Work out the finished part from the listing and answer in its coordinate system (mm). Face numbers are marked on the shaded views. A direction names the side the tool comes from. Give positions to 0.01 mm unless a question says otherwise; leave off trailing zeros. Loops run counter-clockwise (first coordinate to the right, second up) from the corner with the lowest first, then second, coordinate; pieces in that order, holes last. Notation, with made-up numbers: (11.25, -10) - (51.25, -10) arc R17 ccw to (51.25, -6) - close; hole circle Ø9 at (-11, 65.5). An arc over 180 degrees is marked (long way). Use CSV: the item, a comma, the result in double quotes.
from build123d import *

# Parameters (mm, degrees)
SKETCH1_W           = 222.25
SKETCH1_H           = 60.325
BOSS_EXTRUDE1_DEPTH = 25.4
SKETCH2_W           = 12.7
SKETCH2_H           = 60.325
BOSS_EXTRUDE2_DEPTH = 1.5875
SKETCH3_R           = 1.5875
CUT_EXTRUDE1_DEPTH  = 2.5875
SKETCH4_W           = 4.7625
SKETCH4_H           = 19.05
BOSS_EXTRUDE3_DEPTH = 5.08
SKETCH5_W           = 15.875
SKETCH5_H           = 7.9375
BOSS_EXTRUDE4_DEPTH = 12.7
LPATTERN1_COUNT     = 5
LPATTERN1_PITCH     = 22.86
LPATTERN1_COL_COUNT = 5
LPATTERN1_COL_PITCH = 22.86


with BuildPart() as part:
    # Sketch1 → Boss-Extrude1 (new body)
    with BuildSketch(Plane(origin=(0, 0, 0), x_dir=(1, 0, 0), z_dir=(0, 1, 0))):
        with Locations((111.125, 30.1625)):
            Rectangle(SKETCH1_W, SKETCH1_H)
    extrude(amount=BOSS_EXTRUDE1_DEPTH)

    # Sketch2 → Boss-Extrude2 (add)
    with BuildSketch(Plane.XZ):
        with Locations((228.6, -30.1625)):
            Rectangle(SKETCH2_W, SKETCH2_H)
        with Locations((-6.35, -30.1625)):
            Rectangle(SKETCH2_W, SKETCH2_H)
    extrude(amount=-BOSS_EXTRUDE2_DEPTH)

    # Sketch3 → Cut-Extrude1 (cut, through all)
    with BuildSketch(Plane(origin=(0, 1.5875, 0), x_dir=(1, 0, 0), z_dir=(0, 1, 0))):
        with Locations((-7.9375, 46.0375)):
            Circle(SKETCH3_R)
        with Locations((-7.9375, 14.2875)):
            Circle(SKETCH3_R)
        with Locations((230.1875, 14.2875)):
            Circle(SKETCH3_R)
        with Locations((230.1875, 46.0375)):
            Circle(SKETCH3_R)
    extrude(amount=-CUT_EXTRUDE1_DEPTH, mode=Mode.SUBTRACT)

    # Sketch4 → Boss-Extrude3 (add)
    with BuildSketch(Plane(origin=(0, 25.4, 0), x_dir=(1, 0, 0), z_dir=(0, 1, 0))):
        with Locations((111.125, 41.275)):
            Rectangle(SKETCH4_W, SKETCH4_H)
    boss_extrude3 = extrude(amount=BOSS_EXTRUDE3_DEPTH)

    # Sketch5 → Boss-Extrude4 (add)
    with BuildSketch(Plane.XY):
        with Locations((111.125, 13.49375)):
            Rectangle(SKETCH5_W, SKETCH5_H)
    boss_extrude4 = extrude(amount=BOSS_EXTRUDE4_DEPTH)

    # LPattern1: Boss-Extrude3, Boss-Extrude4 ×5
    with Locations(*[(i * LPATTERN1_PITCH, 0, 0) for i in range(1, LPATTERN1_COUNT)]):
        add(boss_extrude3)
        add(boss_extrude4)

    # LPattern1 col: Boss-Extrude3, Boss-Extrude4 ×5
    with Locations(*[(-i * LPATTERN1_COL_PITCH, 0, 0) for i in range(1, LPATTERN1_COL_COUNT)]):
        add(boss_extrude3)
        add(boss_extrude4)


solid = part.part
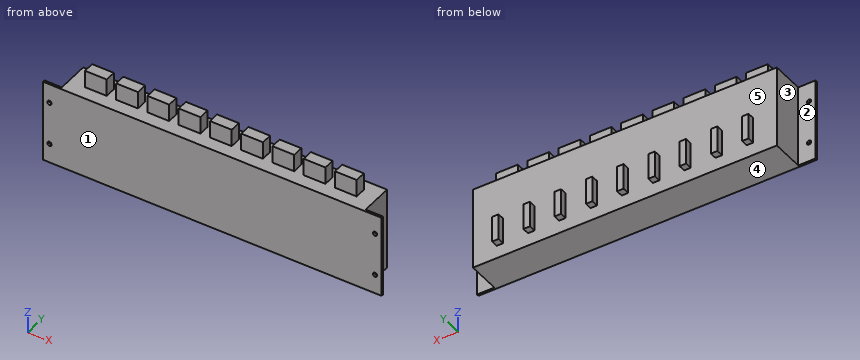
Item 1: A cutting plane is placed at D-D on z = 6. State how many separate pieces and enclosed holes the cut face has, and give its area (3 significant figures).
Determined:
separate pieces,"9"
enclosed holes,"0"
area,"1,130 mm²"
Item 2: A cutting plane is placed at A-A on z = -20.5. Determine the outline of the cut face in (x, y), and give its area (3 significant figures).
Determined:
outline,"(-12.7, 0) - (234.95, 0) - (234.95, 1.59) - (222.25, 1.59) - (222.25, 25.4) - (0, 25.4) - (0, 1.59) - (-12.7, 1.59) - close"
area,"5,690 mm²"
Item 3: For the marked faces 1 and 2, determine the directions among +Z, -Z, +X, -X, +Y, -Y from which every point of the face is accessible in a straight line to the end or side of a thin tool.
Determined:
face 1,"+Z, -Z, +X, -X, -Y"
face 2,"+Z, -Z, -X, +Y"
Item 4: A cutting plane is placed at C-C on y = 4. Determine the outline of the cut face in (x, z) (3 decimals), and give its area (3 significant figures).
Determined:
outline,"(0, -60.325) - (222.25, -60.325) - (222.25, 0) - (0, 0) - close"
area,"13,400 mm²"
Item 5: A cutting plane is placed at B-B on x = 207.5. Determine the outline of the cut face in (y, z) (1 decimal).
Determined:
outline,"(0, -60.3) - (25.4, -60.3) - (25.4, 0) - (17.5, 0) - (17.5, 12.7) - (9.5, 12.7) - (9.5, 0) - (0, 0) - close"
Item 6: Find the intervals of material crossed by line 1 (X direction, y = 20.5, z = -9.5); line 2 (Y direction, x = 27, z = -41); line 3 (Z direction, x = 190, y = 16) (3 decimals), in increasing order.
Determined:
line 1,"x = 0 to 222.25"
line 2,"y = 0 to 25.4"
line 3,"z = -60.325 to 0"
Item 7: Given P1, Ø2.5, axis at y = 27, z = -41, coming from the -X side; P2, Ø10, axis at x = 96, z = -8.5, coming from the +Y side; P3, Ø2.5, axis at y = 15, z = 8.5, coming from the -X side; P4, Ø8, axis at x = 121.5, y = 15.5, coming from the +Z side, each flat-ended and moving along its own axis, determine where each tip first touches the part or whether it passes through.
Determined:
P1,"stops at x = 17.3"
P2,"stops at y = 25.4"
P3,"stops at x = 11.75"
P4,"stops at z = 12.7"
Item 8: The mould has two halves that part along X. Classify the marked faces 3, 4 and 5: pulls with the +X half, pulls with the -X half, needs draft (parallel to the pull), parting line crosses it, or undercut.
Determined:
face 3,"pulls with the -X half"
face 4,"needs draft"
face 5,"undercut"
